Source: CAD feature listing. Evaluate the final solid. Frame: model axes, mm. Face numbers are marked on the shaded views. A direction names the side the tool comes from. Give positions to 0.01 mm unless a question says otherwise; leave off trailing zeros. Order: outer loops, then holes, each group sorted by start corner. A loop starts at its lowest first (then second) coordinate and runs counter-clockwise, first axis right, second up. Notation, with made-up numbers: (81.5, 54) - (115.5, 54) arc R21 cw to (115.5, 64) - close; hole circle Ø7 at (37.25, 23.5). An arc over 180 degrees is marked (long way). One line per item, written item: value. Start each with the question number.
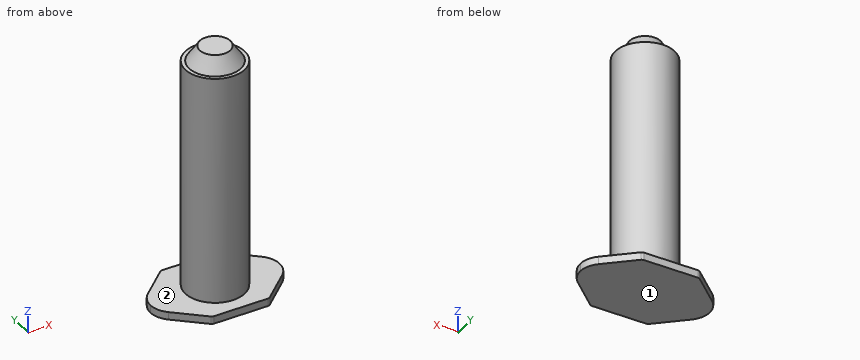
from build123d import *

# Parameters (mm, degrees)
F3_DEPTH = 66.001
F4_R     = 1


with BuildPart() as f1:
    # F0 (on Front) → F1 (revolve)
    with BuildSketch(Plane.XZ):
        Polygon((-17, 0), (0, 0), (0, 66), (-4, 66), (-6.75, 62), (-7.75, 62), (-7.75, 2), (-17, 2), align=None)
    revolve(axis=Axis((0, 0, 33), (0, 0, -1)))

    # F2 (on face) → F3 (cut, through all)
    with BuildSketch(Plane(origin=(0, 0, 0), x_dir=(1, 0, 0), z_dir=(0, 0, -1))):
        with BuildLine():
            Line((-7.5, 11.275), (7.5, 11.275))
            Line((7.5, 11.275), (15, 4.501284))
            ThreePointArc((15, 4.501284), (16.477494, 2.462801), (17, 0))
            ThreePointArc((17, 0), (0, 17), (-17, 0))
            ThreePointArc((-17, 0), (-16.477494, 2.462801), (-15, 4.501284))
            Line((-15, 4.501284), (-7.5, 11.275))
        make_face()
        with BuildLine():
            ThreePointArc((-17, 0), (0, -17), (17, 0))
            ThreePointArc((17, 0), (16.477494, -2.462801), (15, -4.501284))
            Line((15, -4.501284), (7.5, -11.275))
            Line((7.5, -11.275), (-7.5, -11.275))
            Line((-7.5, -11.275), (-15, -4.501284))
            ThreePointArc((-15, -4.501284), (-16.477494, -2.462801), (-17, 0))
        make_face()
    extrude(amount=-F3_DEPTH, mode=Mode.SUBTRACT)

    # F4
    f4_edges = [f1.edges().sort_by_distance(p)[0] for p in [
        (-7.5, -11.275, 1),
        (7.5, -11.275, 1),
        (-7.5, 11.275, 1),
        (7.5, 11.275, 1),
    ]]
    fillet(f4_edges, radius=F4_R)


solid = f1.part
1. Contact query for flat-ended pins moving along their axis: pin 1 Ø6 at (y, z) = (-5, 23.5) entering from +X; pin 2 Ø10 at (x, z) = (6.5, 24.5) entering from +Y; pin 3 Ø3 at (x, y) = (11, 0) entering from +Z. Output: stop coordinate, or through.
2. Section C-C on x = -11. Return the cut outline in (y, z).
3. Ray query, L1, parallel to Z at x = -4, y = 9.75; L2, parallel to Y at x = 4, z = 38.5; L3, parallel to Z at x = -2, y = -6.75. Return the intervals inside material, ascending.
4. Section A-A on x = 0. Return the cut outline in (y, z) (3 decimals).
5. Set-up query: the marked faces 1 and 2. Return all of +Z, -Z, +X, -X, +Y, -Y with unobstructed straight access to the full face (end or side cutting, diameter ignored); none if empty.
6. Section B-B on z = 36.5. Return the cut outline in (x, y), then the cut area to 3 significant figures.
Data:
1. pin 1: stops at x = 7.49
1. pin 2: stops at y = 7.6
1. pin 3: stops at z = 2
2. outline: (-8.11, 0) - (8.11, 0) - (8.11, 2) - (-8.11, 2) - close
3. L1: z = 0 to 2
3. L2: y = -6.64 to 6.64
3. L3: z = 0 to 62
4. outline: (-11.275, 0) - (11.275, 0) - (11.275, 2) - (7.75, 2) - (7.75, 62) - (6.75, 62) - (4, 66) - (-4, 66) - (-6.75, 62) - (-7.75, 62) - (-7.75, 2) - (-11.275, 2) - close
5. face 1: -Z, +X, -X, +Y, -Y
5. face 2: +Z
6. outline: circle Ø15.5 at (0, 0)
6. area: 189 mm2
